Autodesk Inventor part; units mm, degrees
ref_plane "XZ Plane" through (0, 0, 0) normal (0, 1, 0) x (-1, 0, 0)
ref_plane "XY Plane" through (0, 0, 0) normal (0, 0, 1) x (1, 0, 0)
sketch "Sketch1" plane through (0, 0, 0) normal (0, 1, 0) x (-1, 0, 0)
  circle A0 centre (0, 0) radius 25
  dimension "d0" = 50
extrude "Extrusion1" add sketch "Sketch1" along normal blind 490
sketch "Sketch2" plane through (0, 0, 0) normal (0, -1, 0) x (1, 0, 0)
  line L0 (-25, -25) -> (25, -25)
  line L1 (25, -25) -> (25, 25)
  line L2 (25, 25) -> (-25, 25)
  line L3 (-25, 25) -> (-25, -25)
  point P0 (0, 0)
extrude "Extrusion2" add sketch "Sketch2" along normal blind 60
sketch "Sketch3" plane through (0, 0, 0) normal (1, 0, 0) x (0, 1, 0)
  circle A0 centre (-30, 0) radius 15
  line L0 (0, -25) -> (0, 0)
  line L1 (0, 25) -> (-60, 25)
  line L2 (0, -25) -> (-60, -25)
  arc A1 (-30, 25) -> (-30, -25) centre (-30, 0) ccw
  line L3 (-30, 25) -> (-30, 40.1158)
  line L4 (-30, 40.1158) -> (-76.6193, 40.1158)
  line L5 (-76.6193, 40.1158) -> (-77.4473, -45.6375)
  line L6 (-77.4473, -45.6375) -> (-35.1048, -45.6375)
  line L7 (-35.1048, -45.6375) -> (-30, -25)
  dimension "d5" = 30
  dimension "d6" = 30
extrude "Extrusion3" cut sketch "Sketch3" along normal mid plane 100
fillet "Fillet1" radius 24.9775 6 edges at (25, -55, 0) (25, -15, -25) (25, -15, 25) (-25, -55, 0) (-25, -15, -25) (-25, -15, 25)
sketch "Sketch4" plane through (0, 0, 0) normal (1, 0, 0) x (0, 1, 0)
  line L0 (16.2777, 47.2828) -> (16.2777, -82.9386)
  point P0 (0, 0)
properties part number "Piston_Bom"
The listing builds one solid part. Answer for the finished solid, in the listing's coordinates (mm). Round coordinates to 2 decimals unless told otherwise and drop trailing zeros. Write each loop counter-clockwise with the first axis right and the second up, starting at its lowest first coordinate (ties: lowest second). Pieces come first, ordered by that corner, then holes. Notation, with made-up numbers: M -34,29.5 L 13,29.5 A35 cw 13,67.5 Z; hole C 60.5,32 d6. An arc over 180 degrees is marked long. Write each question's results on one line, items separated by ' | '. Start each with the question number.
Item 1: Straight lines are drawn through the part: L1, parallel to Z at x = 0.5, y = -30; L2, parallel to Y at x = 15, z = -6.5; L3, parallel to Z at x = -12, y = -30. For each, find the intervals that lie inside material, in ascending order. Write a range as [from, to].
Item 2: A cutting plane is placed at A-A on y = 268. Write down the section's boundary in (x, z), and give its area (3 significant figures).
Item 3: For a pull along X with two mould halves and no side action, classify faces 1 (the face through (0.35, -16.144, -5.745)), 2 (the face through (-23.846, 241.57, -7.509)), 3 (the face through (14.573, -14.79, -20.324)) as pulls with the +X half, pulls with the -X half, needs draft (parallel to the pull), parting line crosses it, or undercut.
Item 4: Flat-ended cylindrical pins translate along their axes: pin 1 Ø12 at (x, y) = (7, 432) entering from -Z; pin 2 Ø10 at (x, y) = (17, 53) entering from -Z; pin 3 Ø1.5 at (y, z) = (199.5, 15.5) entering from +X; pin 4 Ø18 at (y, z) = (-30, 0) entering from -X. Find the tip coordinate at first contact, or state that the pin passes through.
Check sheet entries:
1) L1: [-25, -15], [15, 25] | L2: [-48.93, -43.52], [-16.48, 490] | L3: [-21.94, -15], [15, 21.94]
2) outline: C 0,0 d50 | area: 1,960 mm²
3) face 1: needs draft | face 2: parting line crosses it | face 3: pulls with the +X half
4) pin 1: z = -24.98 | pin 2: z = -21.93 | pin 3: x = 20.19 | pin 4: through
